Source: CAD feature listing. Evaluate the final solid. Frame: model axes, mm. Face numbers are marked on the shaded views. A direction names the side the tool comes from. Coordinates: 2 decimals unless noted, no trailing zeros. Write each loop counter-clockwise with the first axis right and the second up, starting at its lowest first coordinate (ties: lowest second). Pieces come first, ordered by that corner, then holes. Notation, with made-up numbers: (21, 41) - (26, 41) arc R23 cw to (26, 73) - close; hole circle Ø5 at (-20.75, 75.5). An arc over 180 degrees is marked (long way). One line per question, with ' | ' between items. Start each with the question number.
Q1. Cut plane D-D, the plane z = 21.5. Return loops of the section in (x, y).
Q2. Draft query along X for the marked faces 1, 2, 3 and 4. Return one class per face: +X half, -X half, draft (parallel to the pull), parting line (faces both ways), or undercut.
Q3. Cut plane C-C, the plane x = 0. Return loops of the section in (y, z).
Q4. Access query for the marked faces 5, 6, 7 and 8. Directions: +Z, -Z, +X, -X, +Y, -Y. A direction counts if a zero-diameter tool reaches every point of the face in a straight line with its end or side. Return the directions, or none.
Q5. Line query: line 1 (Y direction, x = 0, z = 17.5); line 2 (Y direction, x = 0, z = 9); line 3 (Z direction, x = -21, y = 5.5). Output: solid intervals per line, ascending.
Q6. Contact query for flat-ended pins moving along their axis: P1, Ø10, axis at y = 0.5, z = 22.5, coming from the +X side; P2, Ø13, axis at x = -28.5, z = 5.5, coming from the +Y side; P3, Ø1.5, axis at x = 6, z = 3.5, coming from the -Y side. Output: stop coordinate, or through.
Q7. Cut plane B-B, the plane z = 10. Return loops of the section in (x, y).
Q8. Cut plane A-A, the plane y = 0. Return loops of the section in (x, z), plus the area to 3 significant figures.
```python
from build123d import *

# Parameters (mm, degrees)
SALIENTE_EXTRUIR1_DEPTH = 12
CROQUIS4_R              = 15
SALIENTE_EXTRUIR2_DEPTH = 14
CROQUIS5_R              = 11
CORTAR_EXTRUIR3_DEPTH   = 18
REDONDEO1_R             = 3
CORTAR_EXTRUIR4_DEPTH   = 8
CORTAR_EXTRUIR6_REACH   = 60.915
CROQUIS2_R              = 5


with BuildPart() as part:
    # Croquis1 → Saliente-Extruir1 (new body)
    with BuildSketch(Plane.XY):
        with BuildLine():
            Line((7.181125002, -21.323260626), (21.213203436, -35.355339059))
            Line((21.213203436, -35.355339059), (35.355339059, -21.213203436))
            Line((35.355339059, -21.213203436), (21.323260626, -7.181125002))
            ThreePointArc((21.323260626, -7.181125002), (8.610377228, 20.787289482), (-20.155644371, 10))
            Line((-20.155644371, 10), (-35, 10))
            ThreePointArc((-35, 10), (-45, 0), (-35, -10))
            Line((-35, -10), (-20.155644371, -10))
            ThreePointArc((-20.155644371, -10), (-8.610377228, -20.787289482), (7.181125002, -21.323260626))
        make_face()
    extrude(amount=SALIENTE_EXTRUIR1_DEPTH)

    # Croquis4 → Saliente-Extruir2 (add)
    with BuildSketch(Plane.XY.offset(12)):
        Circle(CROQUIS4_R)
    extrude(amount=SALIENTE_EXTRUIR2_DEPTH)

    # Croquis5 → Cortar-Extruir3 (cut)
    with BuildSketch(Plane.XY.offset(26)):
        Circle(CROQUIS5_R)
    extrude(amount=-CORTAR_EXTRUIR3_DEPTH, mode=Mode.SUBTRACT)

    # Redondeo1
    redondeo1_edges = [part.edges().sort_by_distance(p)[0] for p in [
        (-15, 0, 12),
    ]]
    fillet(redondeo1_edges, radius=REDONDEO1_R)

    # Croquis3 → Cortar-Extruir4 (cut)
    with BuildSketch(Plane.XY.offset(12)):
        Polygon((31.819805153, -24.748737342), (21.213203436, -14.142135624), (14.142135624, -21.213203436), (24.748737342, -31.819805153), align=None)
    extrude(amount=-CORTAR_EXTRUIR4_DEPTH, mode=Mode.SUBTRACT)

    # Croquis2 → Cortar-Extruir6 (cut, up to next)
    with BuildSketch(Plane.XY.offset(12), mode=Mode.PRIVATE) as cortar_extruir6_sk1:
        with Locations((-35, 0)):
            Circle(CROQUIS2_R)
    cortar_extruir6_tool1 = extrude(cortar_extruir6_sk1.sketch, amount=-CORTAR_EXTRUIR6_REACH, mode=Mode.PRIVATE) & part.part
    add(cortar_extruir6_tool1.solids().sort_by_distance((-35, 0, 12))[0], mode=Mode.SUBTRACT)


solid = part.part
```
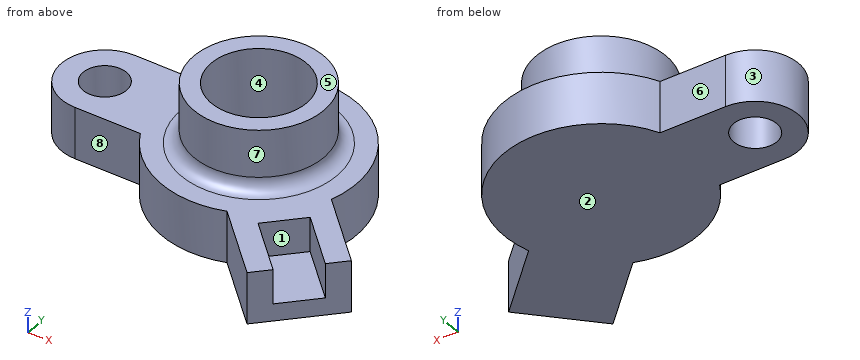
Reply:
1) outline: circle Ø30 at (0, 0); hole circle Ø22 at (0, 0)
2) face 1: undercut | face 2: draft | face 3: -X half | face 4: undercut
3) outline: (-22.5, 0) - (22.5, 0) - (22.5, 12) - (18, 12) arc R3 cw to (15, 15) - (15, 26) - (11, 26) - (11, 8) - (-11, 8) - (-11, 26) - (-15, 26) - (-15, 15) arc R3 cw to (-18, 12) - (-22.5, 12) - close
4) face 5: +Z, +X, -X, +Y, -Y | face 6: +Z, -Z, -X, +Y | face 7: +Z | face 8: +Z, -Z, -X, -Y
5) line 1: y = -15 to -11, 11 to 15 | line 2: y = -22.5 to -11, 11 to 22.5 | line 3: z = 0 to 12
6) P1: stops at x = 15 | P2: stops at y = 10 | P3: stops at y = -21.88
7) outline: (-35, -10) - (-20.16, -10) arc R22.5 ccw to (7.18, -21.32) - (21.21, -35.36) - (24.75, -31.82) - (14.14, -21.21) - (21.21, -14.14) - (31.82, -24.75) - (35.36, -21.21) - (21.32, -7.18) arc R22.5 ccw to (-20.16, 10) - (-35, 10) arc R10 ccw to start; hole circle Ø10 at (-35, 0); hole circle Ø22 at (0, 0)
8) outline: (-45, 0) - (-40, 0) - (-40, 12) - (-45, 12) - close; (-30, 0) - (22.5, 0) - (22.5, 12) - (18, 12) arc R3 cw to (15, 15) - (15, 26) - (11, 26) - (11, 8) - (-11, 8) - (-11, 26) - (-15, 26) - (-15, 15) arc R3 cw to (-18, 12) - (-30, 12) - close | area: 718 mm^2
